For this review, take the finished solid that the model builds, in its own axes (mm). A direction names the side the tool comes from. Coordinates: 2 decimals unless noted, no trailing zeros. Loops run counter-clockwise (first coordinate to the right, second up) from the corner with the lowest first, then second, coordinate; pieces in that order, holes last. Notation, with made-up numbers: (30, 24.25) - (56, 24.25) arc R10 cw to (56, 36.25) - close; hole circle Ø8 at (17.5, -40). An arc over 180 degrees is marked (long way). One line per item, written item: value. Start each with the question number.
1. Take a section at D-D, the plane x = -2.5. State the section outline as (y, z) points, and give its area (3 significant figures).
2. To check wall thickness, follow line 1 (X direction, y = -7, z = 1.5); line 2 (X direction, y = 2.75, z = 3.25); line 3 (Y direction, x = 2.5, z = -3.5). State the ranges of each line that lie inside material, in increasing order. Write a range as from..to.
3. Take a section at B-B, the plane z = 4.5. Count the separate pieces of the cut face and the enclosed holes in it, and give its area (3 significant figures).
4. For faces 1 (the face through (4.409, 3.196, 3.167)), 2 (the face through (-27.881, -0.421, 5.516)), 3 (the face through (-8.409, 3.086, -1.28)), list the 3-axis set-ups (+Z, -Z, +X, -X, +Y, -Y) from which the entire face can be reached by the end or side of a thin tool; tool diameter is ignored.
5. Take a section at A-A, the plane x = -12.5. State the section outline as (y, z) points.
6. The part is to be moulded in two halves that separate along Y. For faces 4 (the face through (5, 5, 2)), 5 (the face through (-29.36, 0, -2)), 6 (the face through (-27.839, -7.493, 0.33)), say which applies: released by +Y, released by -Y, zero draft, split by the parting line, or undercut.
7. Insertion check: pin 1 (2 mm diameter, centred on x = -2.5, z = -2.5, fed in from -Y); pin 2 (2.5 mm diameter, centred on x = 6, y = 5, fed in from +Z); pin 3 (1.2 mm diameter, centred on x = 6.5, z = -5, fed in from +Y); pin 4 (6 mm diameter, centred on y = 1, z = 3.5, fed in from +X). Each pin has a flat end and moves straight along its axis. Give the tip position at first contact, or say it passes through.
```python
from build123d import *

# Parameters (mm, degrees)
CUT_EXTRUDE1_DEPTH = 13
CIRPATTERN1_COUNT  = 4
SKETCH3_R          = 4.5
CUT_EXTRUDE2_DEPTH = 14
CUT_EXTRUDE3_REACH = 42.36
SKETCH4_R          = 1.1
FILLET1_R          = 2


with BuildPart() as part:
    # Sketch1 → Revolve1 (revolve)
    with BuildSketch(Plane.XY):
        Polygon((-4, 7.75), (11, 7.75), (11, 0), (-29.35982328, 0), (-29.35982328, 7.5), (-26.35982328, 7.5), (-26.35982328, 2.5), (-9.25, 2.5), align=None)
    revolve(axis=Axis((0, 0, 0), (1, 0, 0)))

    # Sketch2 → Cut-Extrude1 (cut)
    with BuildSketch(Plane(origin=(11, 0, 0), x_dir=(0, 0, -1), z_dir=(1, 0, 0))):
        with BuildLine():
            Line((-2, 0), (2, 0))
            Line((2, 0), (2, 6.446898479))
            ThreePointArc((2, 6.446898479), (0, 6.75), (-2, 6.446898479))
            Line((-2, 6.446898479), (-2, 0))
        make_face()
    cut_extrude1 = extrude(amount=-CUT_EXTRUDE1_DEPTH, mode=Mode.SUBTRACT)

    # CirPattern1: Cut-Extrude1 ×4 about axis
    cirpattern1_axis = Axis((0, 0, 0), (1, 0, 0))
    for i in range(1, CIRPATTERN1_COUNT):
        add(cut_extrude1.rotate(cirpattern1_axis, i * 360 / CIRPATTERN1_COUNT), mode=Mode.SUBTRACT)

    # Sketch3 → Cut-Extrude2 (cut, through all)
    with BuildSketch(Plane(origin=(-2, 0, 0), x_dir=(0, 0, -1), z_dir=(1, 0, 0))):
        Circle(SKETCH3_R)
    extrude(amount=CUT_EXTRUDE2_DEPTH, mode=Mode.SUBTRACT)

    # Sketch4 → Cut-Extrude3 (cut, up to next)
    with BuildSketch(Plane.ZY.offset(29.35982328), mode=Mode.PRIVATE) as cut_extrude3_sk1:
        with Locations((0, 4.5)):
            Circle(SKETCH4_R)
    cut_extrude3_tool1 = extrude(cut_extrude3_sk1.sketch, amount=-CUT_EXTRUDE3_REACH, mode=Mode.PRIVATE) & part.part
    add(cut_extrude3_tool1.solids().sort_by_distance((-29.359823, 4.5, 0))[0], mode=Mode.SUBTRACT)
    # Sketch4 → Cut-Extrude3 (cut, up to next)
    with BuildSketch(Plane.ZY.offset(29.35982328), mode=Mode.PRIVATE) as cut_extrude3_sk2:
        with Locations((4.5, 0)):
            Circle(SKETCH4_R)
    cut_extrude3_tool2 = extrude(cut_extrude3_sk2.sketch, amount=-CUT_EXTRUDE3_REACH, mode=Mode.PRIVATE) & part.part
    add(cut_extrude3_tool2.solids().sort_by_distance((-29.359823, 0, 4.5))[0], mode=Mode.SUBTRACT)
    # Sketch4 → Cut-Extrude3 (cut, up to next)
    with BuildSketch(Plane.ZY.offset(29.35982328), mode=Mode.PRIVATE) as cut_extrude3_sk3:
        with Locations((0, -4.5)):
            Circle(SKETCH4_R)
    cut_extrude3_tool3 = extrude(cut_extrude3_sk3.sketch, amount=-CUT_EXTRUDE3_REACH, mode=Mode.PRIVATE) & part.part
    add(cut_extrude3_tool3.solids().sort_by_distance((-29.359823, -4.5, 0))[0], mode=Mode.SUBTRACT)
    # Sketch4 → Cut-Extrude3 (cut, up to next)
    with BuildSketch(Plane.ZY.offset(29.35982328), mode=Mode.PRIVATE) as cut_extrude3_sk4:
        with Locations((-4.5, 0)):
            Circle(SKETCH4_R)
    cut_extrude3_tool4 = extrude(cut_extrude3_sk4.sketch, amount=-CUT_EXTRUDE3_REACH, mode=Mode.PRIVATE) & part.part
    add(cut_extrude3_tool4.solids().sort_by_distance((-29.359823, 0, -4.5))[0], mode=Mode.SUBTRACT)

    # Fillet1
    fillet1_edges = [part.edges().sort_by_distance(p)[0] for p in [
        (-9.25, -2.5, 0),
        (-4, -7.75, 0),
    ]]
    fillet(fillet1_edges, radius=FILLET1_R)

    # Sketch5 → Cut-Revolve1 (revolve, cut)
    with BuildSketch(Plane.XY):
        Polygon((-29.35982328, 0), (-24.25982328, 0), (-25.35982328, 1.1), (-29.35982328, 1.1), align=None)
    revolve(axis=Axis((-29.35982328, 0, 0), (-1, 0, 0)), mode=Mode.SUBTRACT)


solid = part.part
```
Solutions:
1. outline: circle Ø15.5 at (0, 0)
1. area: 189 mm2
2. line 1: -29.36..-26.36, -4.59..11
2. line 2: -29.36..-26.36, -7.49..-2
2. line 3: -6.91..-2.83, 2.83..6.91
3. separate pieces: 3
3. enclosed holes: 0
3. area: 192 mm2
4. face 1: +X
4. face 2: -X
4. face 3: none
5. outline: circle Ø5 at (0, 0)
6. face 4: undercut
6. face 5: zero draft
6. face 6: split by the parting line
7. pin 1: y = -7.6
7. pin 2: z = 6.78
7. pin 3: y = 6.38
7. pin 4: x = 11
